Autodesk Inventor part; units mm, degrees
ref_plane "YZ Plane" through (0, 0, 0) normal (1, 0, 0) x (0, 1, 0)
ref_plane "XZ Plane" through (0, 0, 0) normal (0, 1, 0) x (-1, 0, 0)
ref_plane "XY Plane" through (0, 0, 0) normal (0, 0, 1) x (1, 0, 0)
sketch "Sketch1" plane through (0, 0, 0) normal (0, 0, 1) x (1, 0, 0)
  line L0 (0, 0) -> (0, 20)
  line L1 (0, 0) -> (20, 0)
  arc A0 (20, 0) -> (0, 20) centre (0, 0) ccw
  line L2 (0, -4.8284) -> (0, 28.9706)
  dimension "d2" = 20
revolve "Revolution1" add sketch "Sketch1" angle 360 about axis through (0, -10, 0) along (0, 1, 0)
sketch "Sketch4" plane through (0, 0, 0) normal (0, -1, 0) x (1, 0, 0)
  point P0 (0, 0)
  point P1 (0, 0)
hole "Hole2" at (0, 0, 0) direction (0, 1, 0) diameter 3.242 depth 11.8 tip angle 118
shell "Shell2" thickness 4 removed faces 1 at (13.676, 0, 1.6606)
properties part number "Ball_Upper Half" material "Nylon 6/6"
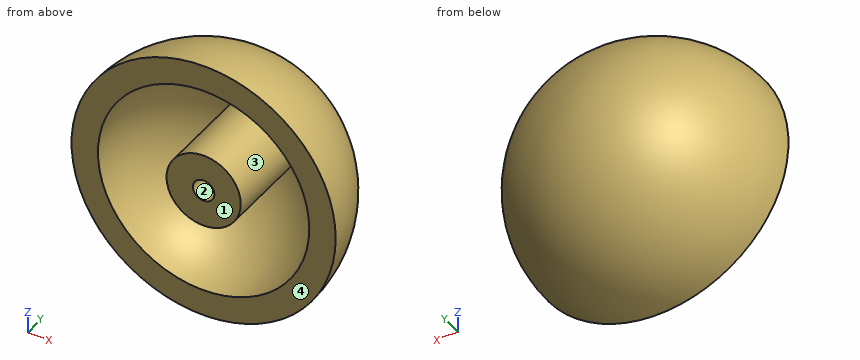
Input: part model. Units: mm. Frame: model coordinates. Face numbers are marked on the shaded views. A direction names the side the tool comes from. Give positions to 0.01 mm unless a question says otherwise; leave off trailing zeros. Order: outer loops, then holes, each group sorted by start corner. A loop starts at its lowest first (then second) coordinate and runs counter-clockwise, first axis right, second up. Notation, with made-up numbers: M 58,71 L 80,71 A19 cw 80,96 Z; hole C 27.25,77 d1. An arc over 180 degrees is marked long. One line per question, with ' | ' between items.
1) Draft query along Z for the marked faces 3 and 4. Return one class per face: pulls with the +Z half, pulls with the -Z half, needs draft (parallel to the pull), parting line crosses it, or undercut.
Filled in:
face 3: undercut | face 4: needs draft
2) Section B-B on z = 10. Output: boundary loops of the cut face in (x, y).
Filled in:
outline: M -17.32,0 L -12.49,0 A12.49 cw 12.49,0 L 17.32,0 A17.32 ccw Z
3) Access query for the marked faces 1 and 2. Directions: +Z, -Z, +X, -X, +Y, -Y. A direction counts if a zero-diameter tool reaches every point of the face in a straight line with its end or side. Return the directions, or none.
Filled in:
face 1: +Z, -Z, +X, -X, -Y | face 2: -Y
4) Contact query for flat-ended pins moving along their axis: P1, Ø3, axis at y = 13, z = -12, coming from the -X side; P2, Ø10, axis at x = -7.5, y = 7.5, coming from the -Z side; P3, Ø12, axis at x = 9, z = -9, coming from the +Y side; P4, Ø4, axis at x = -15.5, z = -2, coming from the -Y side. Output: stop coordinate, or through.
Filled in:
P1: stops at x = -11.74 | P2: stops at z = -19.2 | P3: stops at y = 18.83 | P4: stops at y = 0
5) Section C-C on x = -9. Output: boundary loops of the cut face in (y, z).
Filled in:
outline: M 0,-17.86 A17.86 ccw 0,17.86 L 0,13.23 A13.23 cw 0,-13.23 Z
6) Ray query, L1, parallel to Z at x = 0, y = 8.25; L2, parallel to X at y = 2.5, z = 0; L3, parallel to Z at x = 0, y = 9. Return the intervals inside material, ascending.
Filled in:
L1: z = -18.22 to -13.71, -5.62 to -1.62, 1.62 to 5.62, 13.71 to 18.22 | L2: x = -19.84 to -15.8, -5.62 to -1.62, 1.62 to 5.62, 15.8 to 19.84 | L3: z = -17.86 to -13.23, -5.62 to -1.62, 1.62 to 5.62, 13.23 to 17.86
7) Section A-A on y = 5. Output: boundary loops of the cut face in (x, z).
Filled in:
outline: C 0,0 d38.73; C 0,0 d11.24; hole C 0,0 d30.4; hole C 0,0 d3.24
